Verification items for the finished model (mm, model axes). A direction names the side the tool comes from. Give positions to 0.01 mm unless a question says otherwise; leave off trailing zeros. Loops run counter-clockwise (first coordinate to the right, second up) from the corner with the lowest first, then second, coordinate; pieces in that order, holes last. Notation, with made-up numbers: (57.25, 52) -> (113.25, 52) arc R23 ccw to (113.25, 77) -> close; hole circle Ø5 at (53.25, 18). An arc over 180 degrees is marked (long way). Use one line per item in the form item = value. Start each with the question number.
from build123d import *

# Parameters (mm, degrees)
F1_DEPTH = 3
F2_R     = 5.9
F3_DEPTH = 2
F5_DEPTH = 5
F6_R     = 2.5
F7_DEPTH = 3


with BuildPart() as f1:
    # F0 (on Top) → F1 (new body)
    with BuildSketch(Plane.XY):
        Polygon((-2.44386, -5.9), (2.44386, -5.9), (5.9, -2.44386), (5.9, 2.44386), (2.44386, 5.9), (-2.44386, 5.9), (-5.9, 2.44386), (-5.9, -2.44386), align=None)
        Polygon((-1.615433, -3.9), (-3.9, -1.615433), (-3.9, 1.615433), (-1.615433, 3.9), (1.615433, 3.9), (3.9, 1.615433), (3.9, -1.615433), (1.615433, -3.9), align=None, mode=Mode.SUBTRACT)
    extrude(amount=F1_DEPTH)

    # F2 (on face) → F3 (join)
    with BuildSketch(Plane.XY.offset(3)):
        Circle(F2_R)
    extrude(amount=F3_DEPTH)

    # F4 (on face) → F5 (join)
    with BuildSketch(Plane.XY.offset(5)):
        with BuildLine():
            ThreePointArc((3.872983, 1), (0, 4), (-3.872983, 1))
            Line((-3.872983, 1), (3.872983, 1))
        make_face()
        with BuildLine():
            ThreePointArc((-3.872983, -1), (0, -4), (3.872983, -1))
            Line((3.872983, -1), (-3.872983, -1))
        make_face()
    extrude(amount=F5_DEPTH)

    # F6 (on face) → F7 (join, through all)
    with BuildSketch(Plane(origin=(0, 0, 3), x_dir=(1, 0, 0), z_dir=(0, 0, -1))):
        Circle(F6_R)
    extrude(amount=F7_DEPTH)


solid = f1.part
Item 1: Sectioned sample at A-A, the plane z = 1.25. Enter the section's corners in (x, y).
Item 2: Sectioned sample at C-C, the plane y = 2. Enter the section's corners in (x, z), and give its area (3 significant figures).
Item 3: Draft check along Y on faces 5 (the cylindrical face through (-0.54, 2.44, 1.52)), 6 (the flat face through (0, -1, 7)), 7 (the flat face through (0, -5.9, 1)), 8 (the flat face through (0, 2, 10)). Enter one of: +Y half, -Y half, draft (parallel to the pull), parting line (faces both ways), or undercut.
Item 4: Tool access check on faces 1 (the cylindrical face through (0, -4, 7)), 2 (the flat face through (0, 1, 7)), 3 (the flat face through (-2.774, 2.742, 1.479)), 4 (the flat face through (-2.3, 5.6, 3)). Record the directions out of +Z, -Z, +X, -X, +Y, -Y that give a thin tool (end or side, any length) a straight path to the whole face; none if there is none.
Item 5: Material ranges on line 1 (X direction, y = 0, z = 2.75); line 2 (Y direction, x = -0.5, z = 1); line 3 (Z direction, x = -3, y = 5), recorded low to high.
Item 6: Gauge pin test, flat ends, axial feed: pin 1 Ø1.4 at (x, y) = (1, 5) entering from +Z; pin 2 Ø1 at (y, z) = (-2.5, 7.5) entering from +X. Record the tip position at first contact, or that the pin passes through.
Item 7: Sectioned sample at D-D, the plane z = 8.75. Enter the section's corners in (x, y).
Item 8: Sectioned sample at B-B, the plane x = -4.75. Enter the section's corners in (y, z).
Outcome:
q1.outline = (-5.9, -2.44) -> (-2.44, -5.9) -> (2.44, -5.9) -> (5.9, -2.44) -> (5.9, 2.44) -> (2.44, 5.9) -> (-2.44, 5.9) -> (-5.9, 2.44) -> close; circle Ø5 at (0, 0); hole (-3.9, -1.62) -> (-1.62, -3.9) -> (1.62, -3.9) -> (3.9, -1.62) -> (3.9, 1.62) -> (1.62, 3.9) -> (-1.62, 3.9) -> (-3.9, 1.62) -> close
q2.outline = (-5.9, 0) -> (-3.52, 0) -> (-3.52, 3) -> (-1.5, 3) -> (-1.5, 0) -> (1.5, 0) -> (1.5, 3) -> (3.52, 3) -> (3.52, 0) -> (5.9, 0) -> (5.9, 3) -> (5.55, 3) -> (5.55, 5) -> (3.46, 5) -> (3.46, 10) -> (-3.46, 10) -> (-3.46, 5) -> (-5.55, 5) -> (-5.55, 3) -> (-5.9, 3) -> close
q2.area = 80.2 mm^2
q3.face_5 = undercut
q3.face_6 = undercut
q3.face_7 = -Y half
q3.face_8 = draft
q4.face_1 = +Z, -Y
q4.face_2 = +Z, +X, -X
q4.face_3 = -Z
q4.face_4 = +Z, -X, +Y
q5.line_1 = -5.9 to -3.9, -2.5 to 2.5, 3.9 to 5.9
q5.line_2 = -5.9 to -3.9, -2.45 to 2.45, 3.9 to 5.9
q5.line_3 = 0 to 5
q6.pin_1 = 5
q6.pin_2 = 3.46
q7.outline = (-3.87, -1) arc R4 ccw to (3.87, -1) -> close; (-3.87, 1) -> (3.87, 1) arc R4 ccw to start
q8.outline = (-3.59, 0) -> (3.59, 0) -> (3.59, 3) -> (3.5, 3) -> (3.5, 5) -> (-3.5, 5) -> (-3.5, 3) -> (-3.59, 3) -> close
